Model file for the job. Use its own axes, mm. A direction names the side the tool comes from. Give positions to 0.01 mm unless a question says otherwise; leave off trailing zeros. Order: outer loops, then holes, each group sorted by start corner. A loop starts at its lowest first (then second) coordinate and runs counter-clockwise, first axis right, second up. Notation, with made-up numbers: (47.5, 78) -> (62.5, 78) arc R24 ccw to (62.5, 110) -> close; hole circle Ø1 at (-7, -0.5). An arc over 180 degrees is marked (long way). Use CSV: the item, a comma, the result in double quotes. Start each with the question number.
1. Drop flat-ended pins along their axis: pin 1 (2 mm diameter, centred on x = -128, y = -68, fed in from -Z); pin 2 (1.2 mm diameter, centred on x = -127, z = -6, fed in from -Y); pin 3 (2 mm diameter, centred on x = -127.5, z = 24, fed in from -Y). Give the stop position or say it passes through.
2. 3-axis set-ups, long thin cutter, end or side, ignore diameter. For faces 5 (the flat face through (-127, -72, 0)), 6 (the flat face through (-127, -79, 27.5)), 7 (the flat face through (-127, 75, 22)), 8 (the flat face through (-127, 79, 38)): which of +Z, -Z, +X, -X, +Y, -Y reach the whole face in a straight line?
3. Cut at C-C on y = 67.5. List the corners of the cut face in (x, z), then the cut area to 3 significant figures.
4. Pull direction Y, two halves, no side cores. Call faces 1 (the flat face through (-127, -20, -4)), 2 (the flat face through (-127, 20, -4)), 3 (the flat face through (-127, 60, -4)), 4 (the flat face through (-129, -1, 16)): released by +Y, released by -Y, zero draft, split by the parting line, or undercut.
5. Cut at B-B on x = -127.15. List the corners of the cut face in (y, z).
6. Cut at D-D on z = 20.5. List the corners of the cut face in (x, y), then the cut area to 3 significant figures.
7. Wall check: line 1 (Y direction, x = -127.25, z = -2); line 2 (Y direction, x = -125.65, z = 38.5); line 3 (Z direction, x = -126.25, y = -1.5). Give the ranges that are in metal, low to high. Write a range as from..to.
8. Cut at A-A on z = -2. List the corners of the cut face in (x, y).
```python
from build123d import *

# Parameters (mm, degrees)
SKETCH008_W     = 166
SKETCH008_H     = 48
PAD005_DEPTH    = 4
SKETCH028_W     = 40
SKETCH028_H     = 30
SKETCH028_H_2   = 12
POCKET011_DEPTH = 4.001
SKETCH056_W     = 18
SKETCH056_H     = 10
POCKET022_DEPTH = 4.001


with BuildPart() as part:
    # Sketch008 (on DatumPlane) → Pad005 (new body)
    with BuildSketch(Plane(origin=(-129, 0, -4), x_dir=(0, 1, 0), z_dir=(1, 0, 0))):
        with Locations((0, 20)):
            Rectangle(SKETCH008_W, SKETCH008_H)
    extrude(amount=PAD005_DEPTH)

    # Sketch028 (on Face5 of Pad005) → Pocket011 (cut, through all)
    with BuildSketch(Plane(origin=(-129, 0, -4), x_dir=(0, 1, 0), z_dir=(-1, 0, 0))):
        with Locations((-80, 11)):
            Rectangle(SKETCH028_W, SKETCH028_H)
        with Locations((0, 11)):
            Rectangle(SKETCH028_W, SKETCH028_H)
        with Locations((80, 11)):
            Rectangle(SKETCH028_W, SKETCH028_H)
        with Locations((-95, -25.5)):
            Rectangle(SKETCH028_W, SKETCH028_H_2)
        with Locations((95, -25.5)):
            Rectangle(SKETCH028_W, SKETCH028_H_2)
    extrude(amount=-POCKET011_DEPTH, mode=Mode.SUBTRACT)

    # Sketch056 (on Face4 of Pocket011) → Pocket022 (cut, through all)
    with BuildSketch(Plane(origin=(-129, 0, -4), x_dir=(0, 1, 0), z_dir=(-1, 0, 0))):
        with Locations((70, -45)):
            Rectangle(SKETCH056_W, SKETCH056_H)
    extrude(amount=-POCKET022_DEPTH, mode=Mode.SUBTRACT)


solid = part.part
```
Verdict:
1,pin 1,"z = 0"
1,pin 2,"y = -60"
1,pin 3,"y = -75"
2,face 5,"-Z, +X, -X, -Y"
2,face 6,"+X, -X, -Y"
2,face 7,"+X, -X, +Y"
2,face 8,"+Z, +X, -X"
3,outline,"(-129, 0) -> (-125, 0) -> (-125, 36) -> (-129, 36) -> close"
3,area,"144 mm^2"
4,face 1,"undercut"
4,face 2,"undercut"
4,face 3,"released by +Y"
4,face 4,"zero draft"
5,outline,"(-83, 0) -> (-60, 0) -> (-60, -8) -> (-20, -8) -> (-20, 0) -> (20, 0) -> (20, -8) -> (60, -8) -> (60, 0) -> (83, 0) -> (83, 15.5) -> (75, 15.5) -> (75, 27.5) -> (83, 27.5) -> (83, 40) -> (79, 40) -> (79, 36) -> (61, 36) -> (61, 40) -> (-83, 40) -> (-83, 27.5) -> (-75, 27.5) -> (-75, 15.5) -> (-83, 15.5) -> close"
6,outline,"(-129, -75) -> (-125, -75) -> (-125, 75) -> (-129, 75) -> close"
6,area,"600 mm^2"
7,line 1,"-60..-20, 20..60"
7,line 2,"-83..61, 79..83"
7,line 3,"0..40"
8,outline,"(-129, -60) -> (-125, -60) -> (-125, -20) -> (-129, -20) -> close; (-129, 20) -> (-125, 20) -> (-125, 60) -> (-129, 60) -> close"
